Read the model definition and answer for the solid it produces. Units are mm, in the model's axes. Face numbers are marked on the shaded views. A direction names the side the tool comes from. Round coordinates to 2 decimals unless told otherwise and drop trailing zeros. Order: outer loops, then holes, each group sorted by start corner. A loop starts at its lowest first (then second) coordinate and runs counter-clockwise, first axis right, second up. Notation, with made-up numbers: (-30.5, -16) -> (24.5, -16) arc R23 cw to (24.5, 3) -> close; hole circle Ø3 at (47, -40). An arc over 180 degrees is marked (long way). One line per item, written item: value. Start each with the question number.
1. Section B-B (z = 0) is taken. Give the vertices of the cut face in (x, y).
2. Section A-A (x = 0) is taken. Give the vertices of the cut face in (y, z).
3. Section C-C (y = 1.05) is taken. Give the vertices of the cut face in (x, z).
4. The mould has two halves that part along X. Classify the marked faces 1, 2, 3 and 4: released by +X, released by -X, zero draft, split by the parting line, or undercut.
5. Consider line 1 (X direction, y = 5.5, z = 0); line 2 (Y direction, x = -1, z = -2.75); line 3 (X direction, y = 1.7, z = -0.75). Determine where each line is inside the solid, lowest interval first.
6. Flat-ended cylindrical pins translate along their axes: pin 1 Ø2 at (x, y) = (0, 0.5) entering from -Z; pin 2 Ø1 at (y, z) = (2.5, -2.5) entering from -X; pin 3 Ø2.5 at (y, z) = (5, -3) entering from +X. Find the tip coordinate at first contact, or state that the pin passes through.
7. Section D-D (y = 2.85) is taken. Give the vertices of the cut face in (x, z), then the cut area to 3 significant figures.
8. For the marked faces 5, 6, 7, 8 and 9, determine the directions among +Z, -Z, +X, -X, +Y, -Y from which every point of the face is accessible in a straight line to the end or side of a thin tool.
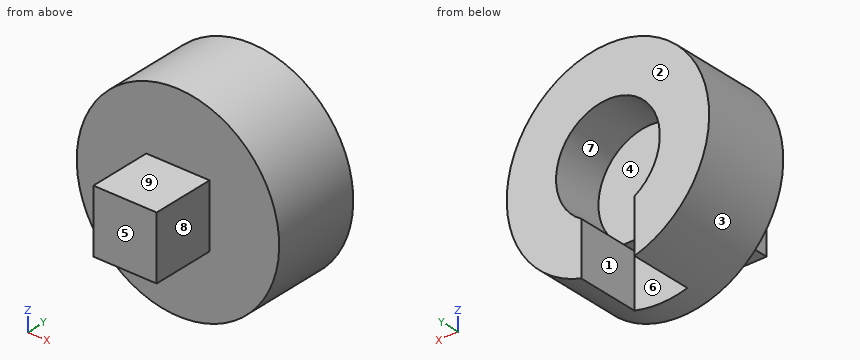
from build123d import *

# Parameters (mm, degrees)
SKETCH1_W           = 2.5
SKETCH1_H           = 2.5
BOSS_EXTRUDE1_DEPTH = 2.5
SKETCH2_R           = 4
BOSS_EXTRUDE2_DEPTH = 3.5
CUT_EXTRUDE1_DEPTH  = 2
CUT_EXTRUDE2_DEPTH  = 0.5


with BuildPart() as part:
    # Sketch1 → Boss-Extrude1 (new body)
    with BuildSketch(Plane(origin=(0, 0, 0), x_dir=(1, 0, 0), z_dir=(0, 1, 0))):
        Rectangle(SKETCH1_W, SKETCH1_H)
    extrude(amount=BOSS_EXTRUDE1_DEPTH)

    # Sketch2 → Boss-Extrude2 (add)
    with BuildSketch(Plane(origin=(0, 2.5, 0), x_dir=(1, 0, 0), z_dir=(0, 1, 0))):
        with Locations(Location((0, 0, 0), (0, 0, 270))):
            Circle(SKETCH2_R)
    extrude(amount=BOSS_EXTRUDE2_DEPTH)

    # Sketch3 → Cut-Extrude1 (cut)
    with BuildSketch(Plane(origin=(0, 6, 0), x_dir=(1, 0, 0), z_dir=(0, 1, 0))):
        with BuildLine():
            Line((1.05, 1.760681686), (1.05, 4))
            Line((1.05, 4), (-1.05, 4))
            Line((-1.05, 4), (-1.05, 1.760681686))
            ThreePointArc((-1.05, 1.760681686), (0, -2.05), (1.05, 1.760681686))
        make_face()
    extrude(amount=-CUT_EXTRUDE1_DEPTH, mode=Mode.SUBTRACT)

    # Sketch5 → Cut-Extrude2 (cut)
    with BuildSketch(Plane(origin=(0, 4, 0), x_dir=(1, 0, 0), z_dir=(0, 1, 0))):
        with BuildLine():
            ThreePointArc((1.05, 1.760681686), (0, 2.05), (-1.05, 1.760681686))
            Line((-1.05, 1.760681686), (1.05, 1.760681686))
        make_face()
        with BuildLine():
            Line((-1.05, 3.85972797), (-1.05, 1.760681686))
            ThreePointArc((-1.05, 1.760681686), (0, 2.05), (1.05, 1.760681686))
            Line((1.05, 1.760681686), (1.05, 3.85972797))
            ThreePointArc((1.05, 3.85972797), (0.5296641, 3.964776909), (-2e-09, 4))
            ThreePointArc((-2e-09, 4), (-0.529664103, 3.964776909), (-1.05, 3.85972797))
        make_face()
    extrude(amount=-CUT_EXTRUDE2_DEPTH, mode=Mode.SUBTRACT)


solid = part.part
Answer:
1. outline: (-4, 2.5) -> (-1.25, 2.5) -> (-1.25, 0) -> (1.25, 0) -> (1.25, 2.5) -> (4, 2.5) -> (4, 6) -> (2.05, 6) -> (2.05, 4) -> (-2.05, 4) -> (-2.05, 6) -> (-4, 6) -> close
2. outline: (0, -1.25) -> (2.5, -1.25) -> (2.5, -4) -> (3.5, -4) -> (3.5, -1.76) -> (4, -1.76) -> (4, 2.05) -> (6, 2.05) -> (6, 4) -> (2.5, 4) -> (2.5, 1.25) -> (0, 1.25) -> close
3. outline: (-1.25, -1.25) -> (1.25, -1.25) -> (1.25, 1.25) -> (-1.25, 1.25) -> close
4. face 1: undercut
4. face 2: zero draft
4. face 3: split by the parting line
4. face 4: undercut
5. line 1: -4 to -2.05, 2.05 to 4
5. line 2: 2.5 to 3.5
5. line 3: -1.25 to 1.25
6. pin 1: z = -1.25
6. pin 2: x = -3.46
6. pin 3: x = 3.6
7. outline: circle Ø8 at (0, 0)
7. area: 50.3 mm^2
8. face 5: +Z, -Z, +X, -X, -Y
8. face 6: -Z, +Y
8. face 7: +Y
8. face 8: +Z, -Z, +X, -Y
8. face 9: +Z, +X, -X, -Y
